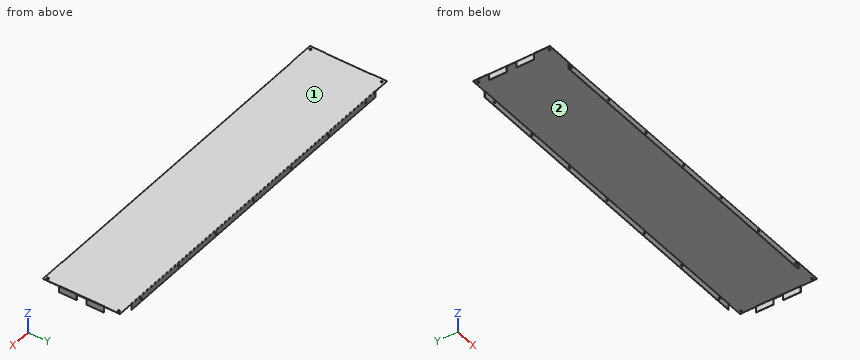
from build123d import *

# Parameters (mm, degrees)
SKETCH_1_W                        = 1140
SKETCH_1_H                        = 238
SM_BASE_FLANGE_1_DEPTH            = 1
SM_EDGE_FLANGE_1_STRIP_W          = 5.4732
SM_EDGE_FLANGE_1_STRIP_H          = 1
SM_EDGE_FLANGE_1_STRIP_CUT_DEPTH  = 138
SM_EDGE_FLANGE_1_RELIEF_W         = 5.9732
SM_EDGE_FLANGE_1_RELIEF_H         = 0.5
SM_EDGE_FLANGE_1_RELIEF_CUT_DEPTH = 1
SM_EDGE_FLANGE_1_DEPTH            = 138
SM_EDGE_FLANGE_1_FLAT_DEPTH       = 1
SM_EDGE_FLANGE_2_STRIP_W          = 5.4732
SM_EDGE_FLANGE_2_STRIP_H          = 1
SM_EDGE_FLANGE_2_STRIP_CUT_DEPTH  = 138
SM_EDGE_FLANGE_2_RELIEF_W         = 5.9732
SM_EDGE_FLANGE_2_RELIEF_H         = 0.5
SM_EDGE_FLANGE_2_RELIEF_CUT_DEPTH = 1
SM_EDGE_FLANGE_2_DEPTH            = 138
SM_EDGE_FLANGE_2_FLAT_DEPTH       = 1
SM_EDGE_FLANGE_3_STRIP_W          = 5.4732
SM_EDGE_FLANGE_3_STRIP_H          = 1
SM_EDGE_FLANGE_3_STRIP_CUT_DEPTH  = 980
SM_EDGE_FLANGE_3_RELIEF_W         = 5.9732
SM_EDGE_FLANGE_3_RELIEF_H         = 0.5
SM_EDGE_FLANGE_3_RELIEF_CUT_DEPTH = 1
SM_EDGE_FLANGE_3_DEPTH            = 980
SM_EDGE_FLANGE_4_STRIP_W          = 5.4732
SM_EDGE_FLANGE_4_STRIP_H          = 1
SM_EDGE_FLANGE_4_STRIP_CUT_DEPTH  = 1040
SM_EDGE_FLANGE_4_RELIEF_W         = 5.9732
SM_EDGE_FLANGE_4_RELIEF_H         = 0.5
SM_EDGE_FLANGE_4_RELIEF_CUT_DEPTH = 1
SM_EDGE_FLANGE_4_DEPTH            = 1040
SKETCH_15_R                       = 3
CUT_EXTRUDE_1_DEPTH               = 619.016181018
SKETCH_18_R                       = 3
CUT_EXTRUDE_2_DEPTH               = 583.599347751


# Sheet-metal steps are written as plain solids
with BuildPart() as part:
    # Sketch 1 → 基体-法兰1 (new body)
    with BuildSketch(Plane.XY):
        Rectangle(SKETCH_1_W, SKETCH_1_H)
    extrude(amount=-SM_BASE_FLANGE_1_DEPTH)

    # 边线-法兰1 strip (across the edge) → 边线-法兰1 strip cut (cut)
    with BuildSketch(Plane(origin=(570, 69, -1), x_dir=(-1, 0, 0), z_dir=(0, -1, 0))):
        with Locations((-1, -0.5)):
            Rectangle(SM_EDGE_FLANGE_1_STRIP_W, SM_EDGE_FLANGE_1_STRIP_H)
    extrude(amount=SM_EDGE_FLANGE_1_STRIP_CUT_DEPTH, mode=Mode.SUBTRACT)

    # 边线-法兰1 relief (on the sheet) → 边线-法兰1 relief cut (cut)
    with BuildSketch(Plane(origin=(568.2634, 69, -1), x_dir=(-1, 0, 0), z_dir=(0, 0, -1))):
        with Locations((-2.4866, 0.25)):
            Rectangle(SM_EDGE_FLANGE_1_RELIEF_W, SM_EDGE_FLANGE_1_RELIEF_H)
        with Locations((-2.4866, -138.25)):
            Rectangle(SM_EDGE_FLANGE_1_RELIEF_W, SM_EDGE_FLANGE_1_RELIEF_H)
    extrude(amount=-SM_EDGE_FLANGE_1_RELIEF_CUT_DEPTH, mode=Mode.SUBTRACT)

    # 边线-法兰1 bend section (across the edge) → 边线-法兰1 (add)
    with BuildSketch(Plane(origin=(570, 69, -1), x_dir=(-1, 0, 0), z_dir=(0, -1, 0))):
        with BuildLine():
            Line((0, 0.7366), (1, 0.7366))
            ThreePointArc((1, 0.7366), (1.215745145, 0.215745145), (1.7366, 0))
            Line((1.7366, 0), (1.7366, -1))
            ThreePointArc((1.7366, -1), (0.508638364, -0.491361636), (0, 0.7366))
        make_face()
    extrude(amount=SM_EDGE_FLANGE_1_DEPTH)

    # 边线-法兰1 profile (on flange) → 边线-法兰1 flat (add)
    with BuildSketch(Plane(origin=(570, 0, -1), x_dir=(0, -1, 0), z_dir=(1, 0, 0))):
        Polygon((-69, 0.7366), (69, 0.7366), (69, 19), (15, 19), (15, 1), (-15, 1), (-15, 19), (-69, 19), align=None)
    extrude(amount=-SM_EDGE_FLANGE_1_FLAT_DEPTH)

    # 边线-法兰2 strip (across the edge) → 边线-法兰2 strip cut (cut)
    with BuildSketch(Plane(origin=(-570, -69, -1), x_dir=(1, 0, 0), z_dir=(0, 1, 0))):
        with Locations((-1, -0.5)):
            Rectangle(SM_EDGE_FLANGE_2_STRIP_W, SM_EDGE_FLANGE_2_STRIP_H)
    extrude(amount=SM_EDGE_FLANGE_2_STRIP_CUT_DEPTH, mode=Mode.SUBTRACT)

    # 边线-法兰2 relief (on the sheet) → 边线-法兰2 relief cut (cut)
    with BuildSketch(Plane(origin=(-568.2634, -69, -1), x_dir=(1, 0, 0), z_dir=(0, 0, -1))):
        with Locations((-2.4866, 0.25)):
            Rectangle(SM_EDGE_FLANGE_2_RELIEF_W, SM_EDGE_FLANGE_2_RELIEF_H)
        with Locations((-2.4866, -138.25)):
            Rectangle(SM_EDGE_FLANGE_2_RELIEF_W, SM_EDGE_FLANGE_2_RELIEF_H)
    extrude(amount=-SM_EDGE_FLANGE_2_RELIEF_CUT_DEPTH, mode=Mode.SUBTRACT)

    # 边线-法兰2 bend section (across the edge) → 边线-法兰2 (add)
    with BuildSketch(Plane(origin=(-570, -69, -1), x_dir=(1, 0, 0), z_dir=(0, 1, 0))):
        with BuildLine():
            Line((0, 0.7366), (1, 0.7366))
            ThreePointArc((1, 0.7366), (1.215745145, 0.215745145), (1.7366, 0))
            Line((1.7366, 0), (1.7366, -1))
            ThreePointArc((1.7366, -1), (0.508638364, -0.491361636), (0, 0.7366))
        make_face()
    extrude(amount=SM_EDGE_FLANGE_2_DEPTH)

    # 边线-法兰2 profile (on flange) → 边线-法兰2 flat (add)
    with BuildSketch(Plane(origin=(-570, 0, -1), x_dir=(0, 1, 0), z_dir=(-1, 0, 0))):
        Polygon((-69, 0.7366), (69, 0.7366), (69, 19), (15, 19), (15, 1), (-15, 1), (-15, 19), (-69, 19), align=None)
    extrude(amount=-SM_EDGE_FLANGE_2_FLAT_DEPTH)

    # 边线-法兰3 strip (across the edge) → 边线-法兰3 strip cut (cut)
    with BuildSketch(Plane(origin=(490, -119, -1), x_dir=(0, 1, 0), z_dir=(-1, 0, 0))):
        with Locations((-1, -0.5)):
            Rectangle(SM_EDGE_FLANGE_3_STRIP_W, SM_EDGE_FLANGE_3_STRIP_H)
    extrude(amount=SM_EDGE_FLANGE_3_STRIP_CUT_DEPTH, mode=Mode.SUBTRACT)

    # 边线-法兰3 relief (on the sheet) → 边线-法兰3 relief cut (cut)
    with BuildSketch(Plane(origin=(490, -117.2634, -1), x_dir=(0, 1, 0), z_dir=(0, 0, -1))):
        with Locations((-2.4866, 0.25)):
            Rectangle(SM_EDGE_FLANGE_3_RELIEF_W, SM_EDGE_FLANGE_3_RELIEF_H)
        with Locations((-2.4866, -980.25)):
            Rectangle(SM_EDGE_FLANGE_3_RELIEF_W, SM_EDGE_FLANGE_3_RELIEF_H)
    extrude(amount=-SM_EDGE_FLANGE_3_RELIEF_CUT_DEPTH, mode=Mode.SUBTRACT)

    # 边线-法兰3 section (across the edge) → 边线-法兰3 (add)
    with BuildSketch(Plane(origin=(490, -119, -1), x_dir=(0, 1, 0), z_dir=(-1, 0, 0))):
        with BuildLine():
            Line((0, 0.7366), (0, 19))
            Line((0, 19), (1, 19))
            Line((1, 19), (1, 0.7366))
            ThreePointArc((1, 0.7366), (1.215745145, 0.215745145), (1.7366, 0))
            Line((1.7366, 0), (1.7366, -1))
            ThreePointArc((1.7366, -1), (0.508638364, -0.491361636), (0, 0.7366))
        make_face()
    extrude(amount=SM_EDGE_FLANGE_3_DEPTH)

    # 边线-法兰4 strip (across the edge) → 边线-法兰4 strip cut (cut)
    with BuildSketch(Plane(origin=(-520, 119, -1), x_dir=(0, -1, 0), z_dir=(1, 0, 0))):
        with Locations((-1, -0.5)):
            Rectangle(SM_EDGE_FLANGE_4_STRIP_W, SM_EDGE_FLANGE_4_STRIP_H)
    extrude(amount=SM_EDGE_FLANGE_4_STRIP_CUT_DEPTH, mode=Mode.SUBTRACT)

    # 边线-法兰4 relief (on the sheet) → 边线-法兰4 relief cut (cut)
    with BuildSketch(Plane(origin=(-520, 117.2634, -1), x_dir=(0, -1, 0), z_dir=(0, 0, -1))):
        with Locations((-2.4866, 0.25)):
            Rectangle(SM_EDGE_FLANGE_4_RELIEF_W, SM_EDGE_FLANGE_4_RELIEF_H)
        with Locations((-2.4866, -1040.25)):
            Rectangle(SM_EDGE_FLANGE_4_RELIEF_W, SM_EDGE_FLANGE_4_RELIEF_H)
    extrude(amount=-SM_EDGE_FLANGE_4_RELIEF_CUT_DEPTH, mode=Mode.SUBTRACT)

    # 边线-法兰4 section (across the edge) → 边线-法兰4 (add)
    with BuildSketch(Plane(origin=(-520, 119, -1), x_dir=(0, -1, 0), z_dir=(1, 0, 0))):
        with BuildLine():
            Line((0, 0.7366), (0, 19))
            Line((0, 19), (1, 19))
            Line((1, 19), (1, 0.7366))
            ThreePointArc((1, 0.7366), (1.215745145, 0.215745145), (1.7366, 0))
            Line((1.7366, 0), (1.7366, -1))
            ThreePointArc((1.7366, -1), (0.508638364, -0.491361636), (0, 0.7366))
        make_face()
    extrude(amount=SM_EDGE_FLANGE_4_DEPTH)

    # 草图15 → 切除-拉伸1 (cut, through all)
    with BuildSketch(Plane.XZ.offset(119)):
        with Locations(Location((-480, -10, 0), (0, 0, 270))):
            Circle(SKETCH_15_R)
        with Locations(Location((-320, -10, 0), (0, 0, 270))):
            Circle(SKETCH_15_R)
        with Locations(Location((-160, -10, 0), (0, 0, 270))):
            Circle(SKETCH_15_R)
        with Locations(Location((0, -10, 0), (0, 0, 270))):
            Circle(SKETCH_15_R)
        with Locations(Location((160, -10, 0), (0, 0, 270))):
            Circle(SKETCH_15_R)
        with Locations(Location((320, -10, 0), (0, 0, 270))):
            Circle(SKETCH_15_R)
        with Locations(Location((480, -10, 0), (0, 0, 270))):
            Circle(SKETCH_15_R)
    extrude(amount=-CUT_EXTRUDE_1_DEPTH, mode=Mode.SUBTRACT)

    # 草图18 → 切除-拉伸2 (cut, through all)
    with BuildSketch(Plane(origin=(0, 0, -1), x_dir=(-1, 0, 0), z_dir=(0, 0, -1))):
        with Locations((-562, -110)):
            Circle(SKETCH_18_R)
        with Locations((-562, 110)):
            Circle(SKETCH_18_R)
        with Locations((560, 110)):
            Circle(SKETCH_18_R)
        with Locations((560, -110)):
            Circle(SKETCH_18_R)
    extrude(amount=-CUT_EXTRUDE_2_DEPTH, mode=Mode.SUBTRACT)


solid = part.part
Work out the finished part from the listing and answer in its coordinate system (mm). Face numbers are marked on the shaded views. Round coordinates to 2 decimals unless told otherwise and drop trailing zeros. Write each loop counter-clockwise with the first axis right and the second up, starting at its lowest first coordinate (ties: lowest second). Pieces come first, ordered by that corner, then holes.
1) The mould has two halves that part along Y. Classify the marked faces 1 and 2: pulls with the +Y half, pulls with the -Y half, needs draft (parallel to the pull), parting line crosses it, or undercut.
2) A cutting plane is placed at B-B (y = 93). Give the vertices of the cut face in (x, z).
3) A cutting plane is placed at A-A (x = -442.5). Give the vertices of the cut face in (y, z), plus the area to 3 significant figures.
4) Given pin 1 Ø6 at (x, y) = (47.5, 59.5) entering from -Z; pin 2 Ø1.1 at (x, z) = (-569.5, -15) entering from +Y; pin 3 Ø1.8 at (y, z) = (-118, -8) entering from -X, each flat-ended and moving along its own axis, determine where each tip first touches the part or whether it passes through.
5) Straight lines are drawn through the part: line 1 (Y direction, x = 175, z = -13.75); line 2 (Z direction, x = 276.5, y = 46); line 3 (X direction, y = 17, z = -4). For each, find the intervals that lie inside material, in ascending order.
Completed:
1. face 1: needs draft
1. face 2: undercut
2. outline: (-570, -1) - (570, -1) - (570, 0) - (-570, 0) - close
3. outline: (-119, -20) - (-118, -20) - (-118, -1.74) arc R0.74 cw to (-117.26, -1) - (117.26, -1) arc R0.74 cw to (118, -1.74) - (118, -20) - (119, -20) - (119, -1.74) arc R1.74 ccw to (117.26, 0) - (-117.26, 0) arc R1.74 ccw to (-119, -1.74) - close
3. area: 275 mm2
4. pin 1: stops at z = -1
4. pin 2: stops at y = 69
4. pin 3: stops at x = -490
5. line 1: y = -119 to -118, 118 to 119
5. line 2: z = -1 to 0
5. line 3: x = -570 to -569, 569 to 570
